Build history of the part. All positions in model axes, mm. Face numbers are marked on the shaded views. A direction names the side the tool comes from. Give positions to 0.01 mm unless a question says otherwise; leave off trailing zeros. Write each loop counter-clockwise with the first axis right and the second up, starting at its lowest first coordinate (ties: lowest second). Pieces come first, ordered by that corner, then holes.
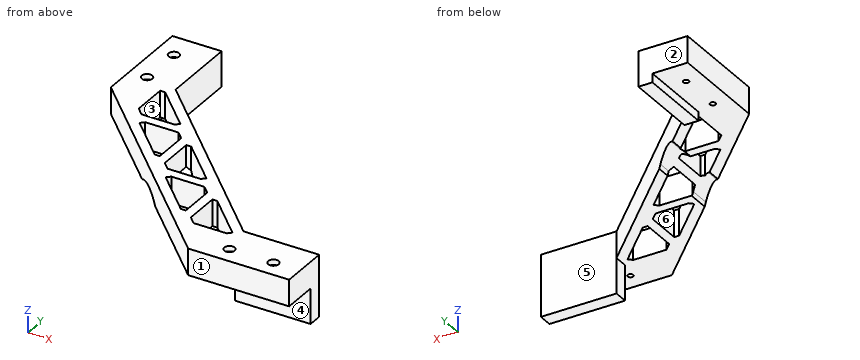
from build123d import *

# Parameters (mm, degrees)
EXTRUDE_1_DEPTH     = 15
SKETCH_3_W          = 43
SKETCH_3_H          = 8
EXTRUDE_2_DEPTH     = 35
SKETCH_4_W          = 8
SKETCH_4_H          = 43
EXTRUDE_3_DEPTH     = 35
CUT_EXTRUDE_1_DEPTH = 244.161454645
SKETCH_6_R          = 1.6
CUT_EXTRUDE_2_DEPTH = 244.161454645
SKETCH_7_R          = 3
CUT_EXTRUDE_3_DEPTH = 3
CHAMFER_1_SIZE      = 2.828427125
CHAMFER_1_SIZE_2    = 4
CUT_EXTRUDE_4_DEPTH = 133
SKETCH_10_W         = 8
SKETCH_10_H         = 15
CUT_EXTRUDE_5_DEPTH = 43


with BuildPart() as part:
    # 草图1 → 凸台-拉伸1 (new body)
    with BuildSketch(Plane.XY):
        Polygon((124.695, -160), (159.695, -160), (159.695, -180), (102.268593129, -180), (-10, -67.731406871), (-10, -10.305), (10, -10.305), (10, -45.305), align=None)
    extrude(amount=EXTRUDE_1_DEPTH)

    # 草图3 → 凸台-拉伸2 (add)
    with BuildSketch(Plane.XY.offset(15)):
        with Locations((138.195, -156)):
            Rectangle(SKETCH_3_W, SKETCH_3_H)
    extrude(amount=-EXTRUDE_2_DEPTH)

    # 草图4 → 凸台-拉伸3 (add)
    with BuildSketch(Plane.XY.offset(15)):
        with Locations((14, -31.805)):
            Rectangle(SKETCH_4_W, SKETCH_4_H)
    extrude(amount=-EXTRUDE_3_DEPTH)

    # 草图5 → 切除-拉伸1 (cut, through all)
    with BuildSketch(Plane.XY.offset(15)):
        Polygon((50.023383861, -93.106558454), (50.023383861, -119.976616139), (76.893441546, -119.976616139), align=None)
        Polygon((55.523383861, -125.476616139), (82.393441546, -125.476616139), (82.393441546, -152.346673824), align=None)
        Polygon((12.153326176, -55.236500769), (12.153326176, -82.106558454), (39.023383861, -82.106558454), align=None)
        Polygon((87.893441546, -130.976616139), (87.893441546, -157.846673824), (114.763499231, -157.846673824), align=None)
        Polygon((17.653326176, -87.606558454), (44.523383861, -87.606558454), (44.523383861, -114.476616139), align=None)
    extrude(amount=-CUT_EXTRUDE_1_DEPTH, mode=Mode.SUBTRACT)

    # 草图6 → 切除-拉伸2 (cut, through all)
    with BuildSketch(Plane.XY.offset(15)):
        with Locations((0, -50.305)):
            Circle(SKETCH_6_R)
        with Locations((0, -25.305)):
            Circle(SKETCH_6_R)
        with Locations((119.695, -170)):
            Circle(SKETCH_6_R)
        with Locations((144.695, -170)):
            Circle(SKETCH_6_R)
    extrude(amount=-CUT_EXTRUDE_2_DEPTH, mode=Mode.SUBTRACT)

    # 草图7 → 切除-拉伸3 (cut)
    with BuildSketch(Plane.XY.offset(15)):
        with Locations((0, -25.305)):
            Circle(SKETCH_7_R)
        with Locations((0, -50.305)):
            Circle(SKETCH_7_R)
        with Locations((119.695, -170)):
            Circle(SKETCH_7_R)
        with Locations((144.695, -170)):
            Circle(SKETCH_7_R)
    extrude(amount=-CUT_EXTRUDE_3_DEPTH, mode=Mode.SUBTRACT)

    # 倒角1
    # the kernel refuses this chamfer: 4, 2.828427125 mm, written as the material it adds along each edge
    with BuildSketch(Plane(origin=(82.393441546, -152.346673824, 15), x_dir=(0.05647824947248942, 0.9984038297885898, 0), z_dir=(0, 0, -1)), Plane(origin=(55.523383861, -125.476616139, 15), x_dir=(0.6660419652145875, -0.7459142715976752, 0), z_dir=(0, 0, -1)), Plane(origin=(87.893441546, -130.976616139, 15), x_dir=(-0.05647824947248942, -0.9984038297885898, 0), z_dir=(0, 0, -1)), Plane(origin=(12.153326176, -55.236500769, 15), x_dir=(-0.05647824947249038, -0.9984038297885897, 0), z_dir=(0, 0, -1)), Plane(origin=(44.523383861, -114.476616139, 15), x_dir=(0.05647824947248914, 0.9984038297885898, 0), z_dir=(0, 0, -1)), Plane(origin=(17.653326176, -87.606558454, 15), x_dir=(0.6660419652145882, -0.7459142715976745, 0), z_dir=(0, 0, -1)), Plane(origin=(50.023383861, -93.106558454, 15), x_dir=(-0.05647824947248914, -0.9984038297885898, 0), z_dir=(0, 0, -1))) as chamfer_1_piece_1:
        Polygon((CHAMFER_1_SIZE * 0.998403829699, -CHAMFER_1_SIZE * 0.0564782494674), (CHAMFER_1_SIZE_2 * 0.666041965215, -CHAMFER_1_SIZE_2 * 0.745914271598), (0, 0), align=None)
    extrude(amount=15)
    with BuildSketch(Plane(origin=(82.393441546, -125.476616139, 15), x_dir=(0.02749587661058555, -0.9996219169112968, 0), z_dir=(0, 0, -1)), Plane(origin=(87.893441546, -157.846673824, 15), x_dir=(-0.02749587661058555, 0.9996219169112968, 0), z_dir=(0, 0, -1)), Plane(origin=(12.153326176, -82.106558454, 15), x_dir=(-0.02749587661058651, 0.9996219169112968, 0), z_dir=(0, 0, -1)), Plane(origin=(44.523383861, -87.606558454, 15), x_dir=(0.027495876610585647, -0.9996219169112968, 0), z_dir=(0, 0, -1)), Plane(origin=(50.023383861, -119.976616139, 15), x_dir=(-0.027495876610585647, 0.9996219169112968, 0), z_dir=(0, 0, -1))) as chamfer_1_piece_2:
        Polygon((CHAMFER_1_SIZE_2 * 0.999621916911, CHAMFER_1_SIZE_2 * 0.0274958766106), (-CHAMFER_1_SIZE_2 * 0.0274958766106, CHAMFER_1_SIZE_2 * 0.999621916911), (0, 0), align=None)
    extrude(amount=15)
    with BuildSketch(Plane(origin=(114.763499231, -157.846673824, 15), x_dir=(-0.9996219169112968, -0.0274958766105891, 0), z_dir=(0, 0, -1)), Plane(origin=(39.023383861, -82.106558454, 15), x_dir=(-0.9996219169112968, -0.027495876610585647, 0), z_dir=(0, 0, -1)), Plane(origin=(76.893441546, -119.976616139, 15), x_dir=(-0.9996219169112968, -0.027495876610585647, 0), z_dir=(0, 0, -1))) as chamfer_1_piece_3:
        Polygon((CHAMFER_1_SIZE_2 * 0.999621916911, CHAMFER_1_SIZE_2 * 0.0274958766106), (CHAMFER_1_SIZE * 0.687396915203, CHAMFER_1_SIZE * 0.726281956812), (0, 0), align=None)
    extrude(amount=15)

    # 草图9 → 切除-拉伸4 (cut)
    with BuildSketch(Plane(origin=(0, -10.305, 0), x_dir=(1, 0, 0), z_dir=(0, 1, 0))):
        with BuildLine():
            Line((54.586563641, 0), (35.413436359, 0))
            Line((35.413436359, 0), (37.089053206, -1.18512051))
            ThreePointArc((37.089053206, -1.18512051), (45, -3.7), (52.910946794, -1.18512051))
            Line((52.910946794, -1.18512051), (54.586563641, 0))
        make_face()
    extrude(amount=-CUT_EXTRUDE_4_DEPTH, mode=Mode.SUBTRACT)

    # 草图10 → 切除-拉伸5 (cut)
    with BuildSketch(Plane(origin=(0, -10.305, 0), x_dir=(1, 0, 0), z_dir=(0, 1, 0))):
        with Locations((14, 12.5)):
            Rectangle(SKETCH_10_W, SKETCH_10_H)
    extrude(amount=-CUT_EXTRUDE_5_DEPTH, mode=Mode.SUBTRACT)


solid = part.part
1. Saw through at C-C on y = -162. Give the cut face in (x, z) (3 decimals), plus the area to 3 significant figures.
2. Drill centre lines: line 1 along X through (y, z) = (-143, 4.5) (3 decimals); line 2 along Y through (x, z) = (0, 5) (3 decimals); line 3 along X through (y, z) = (-170, 14.15) (3 decimals). Where is each one in solid material? Low to high.
3. 3-axis set-ups, long thin cutter, end or side, ignore diameter. For the marked faces 4, 5 and 6: which of +Z, -Z, +X, -X, +Y, -Y reach the whole face in a straight line?
4. Saw through at A-A on y = -140. Give the cut face in (x, z) (3 decimals), plus the area to 3 significant figures.
5. Drop flat-ended pins along their axis: pin 1 (3.5 mm diameter, centred on x = 144.695, y = -170, fed in from +Z); pin 2 (5 mm diameter, centred on x = 144.695, y = -170, fed in from -Z); pin 3 (4 mm diameter, centred on y = -155.5, z = -9, fed in from -X) (3 decimals). Give the stop position or say it passes through.
6. Mould opens along Y. For the marked faces 1, 2 and 3 say: pulls with the +Y half, pulls with the -Y half, needs draft (parallel to the pull), parting line crosses it, or undercut.
7. Saw through at B-B on z = -10. Give the cut face in (x, y) (3 decimals), plus the area to 3 significant figures.
Outcome:
1. outline: (84.269, 0) - (159.695, 0) - (159.695, 15) - (84.269, 15) - close
1. area: 1,130 mm2
2. line 1: x = 65.269 to 73.047, 82.393 to 87.893, 99.917 to 107.695
2. line 2: y = -77.731 to -51.905, -48.705 to -26.905, -23.705 to -10.305
2. line 3: x = 92.269 to 116.695, 122.695 to 141.695, 147.695 to 159.695
3. face 4: -Z, +X, -X, -Y
3. face 5: +Z, -Z, +X, +Y
3. face 6: +Z, -Z
4. outline: (62.269, 0) - (70.047, 0) - (70.047, 15) - (62.269, 15) - close; (82.393, 0) - (87.893, 0) - (87.893, 15) - (82.393, 15) - close; (96.917, 0) - (104.695, 0) - (104.695, 15) - (96.917, 15) - close
4. area: 316 mm2
5. pin 1: stops at z = 12
5. pin 2: stops at z = 0
5. pin 3: stops at x = 116.695
6. face 1: pulls with the -Y half
6. face 2: pulls with the +Y half
6. face 3: undercut
7. outline: (116.695, -160) - (159.695, -160) - (159.695, -152) - (116.695, -152) - close
7. area: 344 mm2
